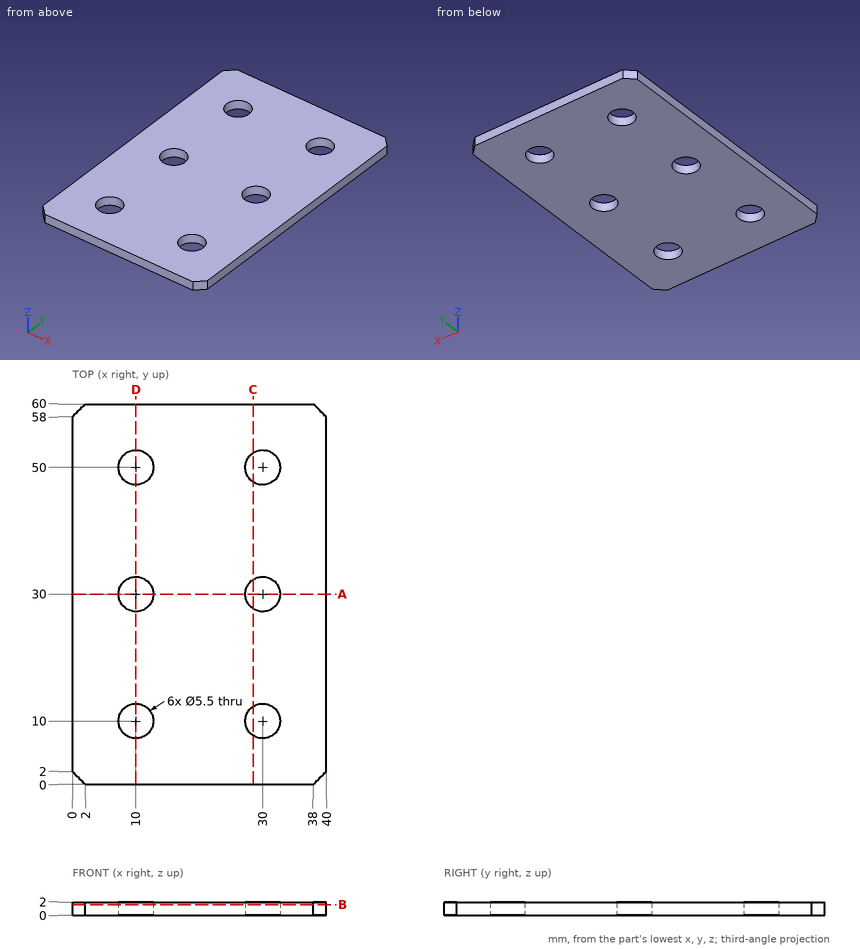
Geometry check sheet. Reference: drawing and pictorial views, mm from the part's lowest x, y, z. Round coordinates to 2 decimals unless told otherwise and drop trailing zeros. Loops run counter-clockwise (first coordinate to the right, second up) from the corner with the lowest first, then second, coordinate; pieces in that order, holes last. Notation, with made-up numbers: M 68.5,51.5 L 81.5,51.5 A20 ccw 81.5,69.5 Z; hole C 66.5,15.25 d11. An arc over 180 degrees is marked long. Return JSON: item names as keys, results as strings. Group by question number.
(1) Scan lines: line 1 along Y through (x, z) = (30, 0.75); line 2 along Y through (x, z) = (32, 0.3). Record each from-to range of solid material in increasing order. Write a range as [from, to].
(2) Section check B-B, the plane z = 1.65. Enter the section's corners in (x, y), and give its area (3 significant figures).
(3) Go/stop test with a flat-tipped pin: pin 1 (3.5 mm diameter, centred on x = 10, y = 10, fed in from +Z). Record where the tip stops, or that it passes through.
(4) Section check A-A, the plane y = 30. Enter the section's corners in (x, z), and give its area (3 significant figures).
(5) Section check D-D, the plane x = 10. Enter the section's corners in (y, z), and give its area (3 significant figures).
(6) Section check C-C, the plane x = 28.5. Enter the section's corners in (y, z).
Data:
{
 "1": {"line 1": "[0, 7.25], [12.75, 27.25], [32.75, 47.25], [52.75, 60]", "line 2": "[0, 8.11], [11.89, 28.11], [31.89, 48.11], [51.89, 60]"},
 "2": {"outline": "M 0,2 L 2,0 L 38,0 L 40,2 L 40,58 L 38,60 L 2,60 L 0,58 Z; hole C 10,10 d5.5; hole C 10,30 d5.5; hole C 10,50 d5.5; hole C 30,10 d5.5; hole C 30,30 d5.5; hole C 30,50 d5.5", "area": "2,250 mm²"},
 "3": {"pin 1": "through"},
 "4": {"outline": "M 0,0 L 7.25,0 L 7.25,2 L 0,2 Z; M 12.75,0 L 27.25,0 L 27.25,2 L 12.75,2 Z; M 32.75,0 L 40,0 L 40,2 L 32.75,2 Z", "area": "58.0 mm²"},
 "5": {"outline": "M 0,0 L 7.25,0 L 7.25,2 L 0,2 Z; M 12.75,0 L 27.25,0 L 27.25,2 L 12.75,2 Z; M 32.75,0 L 47.25,0 L 47.25,2 L 32.75,2 Z; M 52.75,0 L 60,0 L 60,2 L 52.75,2 Z", "area": "87.0 mm²"},
 "6": {"outline": "M 0,0 L 7.7,0 L 7.7,2 L 0,2 Z; M 12.3,0 L 27.7,0 L 27.7,2 L 12.3,2 Z; M 32.3,0 L 47.7,0 L 47.7,2 L 32.3,2 Z; M 52.3,0 L 60,0 L 60,2 L 52.3,2 Z"}
}
